```python
from build123d import *

# Parameters (mm, degrees)
SKETCH1_R           = 49.5046
BOSS_EXTRUDE1_DEPTH = 5.08
SKETCH2_R           = 47.625
BOSS_EXTRUDE2_DEPTH = 3.175
SKETCH3_R           = 6.731
SKETCH3_R_2         = 3.96875
SKETCH3_R_3         = 9.525
CUT_EXTRUDE1_DEPTH  = 9.255
SKETCH7_R           = 65.421404769
CUT_EXTRUDE3_DEPTH  = 5.08
SKETCH9_R           = 11.176
CUT_EXTRUDE5_DEPTH  = 0.762


with BuildPart() as part:
    # Sketch1 → Boss-Extrude1 (new body)
    with BuildSketch(Plane.XY):
        Circle(SKETCH1_R)
    extrude(amount=BOSS_EXTRUDE1_DEPTH)

    # Sketch2 → Boss-Extrude2 (add)
    with BuildSketch(Plane.XY.offset(5.08)):
        Circle(SKETCH2_R)
    extrude(amount=BOSS_EXTRUDE2_DEPTH)

    # Sketch3 → Cut-Extrude1 (cut, through all)
    with BuildSketch(Plane.XY.offset(8.255)):
        with Locations((-12.7, -31.166793627)):
            Circle(SKETCH3_R)
        with Locations((12.7, -31.166793627)):
            Circle(SKETCH3_R)
        with Locations((-36.83, 0)):
            Circle(SKETCH3_R_2)
        with Locations((36.83, 0)):
            Circle(SKETCH3_R_2)
        Circle(SKETCH3_R_3)
    extrude(amount=-CUT_EXTRUDE1_DEPTH, mode=Mode.SUBTRACT)

    # Sketch7 → Cut-Extrude3 (cut)
    with BuildSketch(Plane(origin=(0, 0, 0), x_dir=(-1, 0, 0), z_dir=(0, 0, -1))):
        Circle(SKETCH7_R)
    extrude(amount=-CUT_EXTRUDE3_DEPTH, mode=Mode.SUBTRACT)

    # Sketch9 → Cut-Extrude5 (cut)
    with BuildSketch(Plane.XY.offset(8.255)):
        with Locations((-12.7, -31.166793627)):
            Circle(SKETCH9_R)
        with Locations((12.7, -31.166793627)):
            Circle(SKETCH9_R)
    extrude(amount=-CUT_EXTRUDE5_DEPTH, mode=Mode.SUBTRACT)


solid = part.part
```
Geometry: final body of the model. Coordinates: model frame, mm. A direction names the side the tool comes from. Coordinates: 2 decimals unless noted, no trailing zeros. Write each loop counter-clockwise with the first axis right and the second up, starting at its lowest first coordinate (ties: lowest second). Pieces come first, ordered by that corner, then holes. Notation, with made-up numbers: M 40.25,45 L 92.25,45 A32 cw 92.25,80 Z; hole C -27.5,53 d3. An arc over 180 degrees is marked long. Answer as CSV lines item,"result". Start each with the question number.
Q1. Cut plane A-A on y = 0. Return the cut outline in (x, z) (3 decimals), then the cut area to 3 significant figures.
Q2. Cut plane C-C on z = 6.85. Count the separate pieces of the cut face and the enclosed holes in it, then the cut area to 3 significant figures.
Q3. Cut plane B-B on x = 0. Return the cut outline in (y, z) (3 decimals).
Q4. Line query: line 1 (Y direction, x = 0, z = 6.7) (3 decimals); line 2 (Y direction, x = 7, z = 5.75); line 3 (Y direction, x = -18, z = 6.9). Output: solid intervals per line, ascending. Write a range as from..to.
Q5. Cut plane D-D on x = 12.7. Return the cut outline in (y, z) (3 decimals).
Q6. Pin query (flat end, axial travel): P1, Ø7, axis at x = -36.83, y = 0, coming from the +Z side; P2, Ø11, axis at x = 9, y = -28, coming from the +Z side. Return the tip coordinate at first contact, or that it passes through.
Q7. Reachability of faces 1 (the cylindrical face through (-15.123, -42.077, 7.879)), 2 (the cylindrical face through (-13.576, -24.493, 6.303)) from +Z, -Z, +X, -X, +Y, -Y: full face, straight path, thin tool, end or side. Return the list, or none.
Q8. Mould query, pull axis X, two halves, no side actions, for faces 3 (the cylindrical face through (-7.559, -5.796, 6.69)), 4 (the flat face through (-10, 1, 5.08)), 5 (the cylindrical face through (-37.794, -28.979, 6.645)). Classes: released by +X, released by -X, zero draft, split by the parting line, or undercut.
Findings below:
1,outline,"M -47.625,5.08 L -40.799,5.08 L -40.799,8.255 L -47.625,8.255 Z; M -32.861,5.08 L -9.525,5.08 L -9.525,8.255 L -32.861,8.255 Z; M 9.525,5.08 L 32.861,5.08 L 32.861,8.255 L 9.525,8.255 Z; M 40.799,5.08 L 47.625,5.08 L 47.625,8.255 L 40.799,8.255 Z"
1,area,"192 mm2"
2,separate pieces,"1"
2,enclosed holes,"5"
2,area,"6,460 mm2"
3,outline,"M -47.625,5.08 L -9.525,5.08 L -9.525,8.255 L -47.625,8.255 Z; M 9.525,5.08 L 47.625,5.08 L 47.625,8.255 L 9.525,8.255 Z"
4,line 1,"y = -47.625..-9.525, 9.525..47.625"
4,line 2,"y = -47.11..-34.75, -27.59..-6.46, 6.46..47.11"
4,line 3,"y = -44.09..-35.32, -27.02..44.09"
5,outline,"M -45.9,5.08 L -37.898,5.08 L -37.898,7.493 L -42.343,7.493 L -42.343,8.255 L -45.9,8.255 Z; M -24.436,5.08 L 45.9,5.08 L 45.9,8.255 L -19.991,8.255 L -19.991,7.493 L -24.436,7.493 Z"
6,P1,"passes through"
6,P2,"stops at z = 7.49"
7,face 1,"+Z"
7,face 2,"+Z, -Z"
8,face 3,"undercut"
8,face 4,"zero draft"
8,face 5,"split by the parting line"
